For this review, take the finished solid that the model builds, in its own axes (mm). Face numbers are marked on the shaded views. A direction names the side the tool comes from. Coordinates: 2 decimals unless noted, no trailing zeros. Write each loop counter-clockwise with the first axis right and the second up, starting at its lowest first coordinate (ties: lowest second). Pieces come first, ordered by that corner, then holes.
```python
from build123d import *

# Parameters (mm, degrees)
SKETCH1_W           = 56.642
SKETCH1_H           = 32.258
BOSS_EXTRUDE1_DEPTH = 30.48
SHELL1_T            = -2.54
BOSS_EXTRUDE2_DEPTH = 6.35
FILLET2_R           = 2.54
FILLET3_R           = 2.54
CUT_EXTRUDE9_REACH  = 54.647
SKETCH10_W          = 22.86
SKETCH10_H          = 2.032
BOSS_EXTRUDE3_REACH = 46.623
SKETCH13_W          = 2.54
SKETCH13_H          = 3.81
SKETCH14_W          = 3.81
SKETCH14_H          = 1.27
BOSS_EXTRUDE4_DEPTH = 25.4
CUT_EXTRUDE10_DEPTH = 2.54
CUT_EXTRUDE11_REACH = 46.623
SKETCH16_W          = 9.652
SKETCH16_H          = 4.826
SKETCH11_R          = 1.27
CUT_EXTRUDE12_DEPTH = 9.398
MIRROR2_START       = 4.572
MIRROR2_OUTLINE_W   = 25.4
MIRROR2_OUTLINE_H   = 3.81
MIRROR2_DEPTH       = 2.54
SKETCH17_W          = 2.54
SKETCH17_H          = 3.81
CUT_EXTRUDE13_DEPTH = 23.368
SKETCH18_W          = 7.2898
SKETCH18_H          = 2.54
CUT_EXTRUDE14_DEPTH = 7.366
FILLET4_R           = 1.27
SKETCH19_W          = 2.54
SKETCH19_H          = 5.08
BOSS_EXTRUDE5_DEPTH = 2.54
CUT_EXTRUDE15_START = -23.368
SKETCH20_W          = 2.54
SKETCH20_H          = 3.81
CUT_EXTRUDE15_DEPTH = 23.368
SKETCH22_W          = 2.657331224
SKETCH22_H          = 5.08
CUT_EXTRUDE18_DEPTH = 6.858
SKETCH23_W          = 2.581688451
SKETCH23_H          = 6.7056
CUT_EXTRUDE19_DEPTH = 6.858
SKETCH24_W          = 4.254264989
SKETCH24_H          = 4.461970644
CUT_EXTRUDE20_DEPTH = 7.112


# Read off the part's stored shape, not the designer's step: Mirror2
with BuildPart() as part:
    # Sketch1 → Boss-Extrude1 (new body)
    with BuildSketch(Plane(origin=(0, 0, 0), x_dir=(1, 0, 0), z_dir=(0, 1, 0))):
        Rectangle(SKETCH1_W, SKETCH1_H)
    extrude(amount=BOSS_EXTRUDE1_DEPTH)

    # Shell1
    shell1_openings = [part.faces().sort_by_distance(p)[0] for p in [
        (0, 30.48, 0),
    ]]
    offset(amount=SHELL1_T, openings=shell1_openings, kind=Kind.INTERSECTION)

    # Sketch3 → Boss-Extrude2 (add)
    with BuildSketch(Plane(origin=(0, 30.48, 0), x_dir=(1, 0, 0), z_dir=(0, 1, 0))):
        with BuildLine():
            Line((-25.781, 13.589), (-25.781, 6.35))
            Line((-25.781, 6.35), (-23.9268, 6.35))
            ThreePointArc((-23.9268, 6.35), (-22.543840557, 6.922840557), (-21.971, 8.3058))
            Line((-21.971, 8.3058), (-21.971, 13.589))
            Line((-21.971, 13.589), (-25.781, 13.589))
        make_face()
        with BuildLine():
            Line((-21.971, -13.589), (-21.971, -8.3058))
            ThreePointArc((-21.971, -8.3058), (-22.543840557, -6.922840557), (-23.9268, -6.35))
            Line((-23.9268, -6.35), (-25.781, -6.35))
            Line((-25.781, -6.35), (-25.781, -13.589))
            Line((-25.781, -13.589), (-21.971, -13.589))
        make_face()
        with BuildLine():
            Line((25.781, 13.589), (19.2532, 13.589))
            Line((19.2532, 13.589), (19.2532, 5.969))
            ThreePointArc((19.2532, 5.969), (19.625174388, 5.070974388), (20.5232, 4.699))
            Line((20.5232, 4.699), (25.781, 4.699))
            Line((25.781, 4.699), (25.781, 13.589))
        make_face()
        with BuildLine():
            Line((25.781, -4.699), (25.781, -13.589))
            Line((25.781, -13.589), (19.2532, -13.589))
            Line((19.2532, -13.589), (19.2532, -5.969))
            ThreePointArc((19.2532, -5.969), (19.625174388, -5.070974388), (20.5232, -4.699))
            Line((20.5232, -4.699), (25.781, -4.699))
        make_face()
    extrude(amount=-BOSS_EXTRUDE2_DEPTH)

    # Fillet2
    fillet2_edges = [part.edges().sort_by_distance(p)[0] for p in [
        (28.321, 15.24, 16.129),
        (-28.321, 15.24, 16.129),
        (-28.321, 15.24, -16.129),
        (28.321, 15.24, -16.129),
    ]]
    fillet(fillet2_edges, radius=FILLET2_R)

    # Fillet3
    fillet3_edges = [part.edges().sort_by_distance(p)[0] for p in [
        (-25.781, 24.13, 9.9695),
        (-23.876, 24.13, 13.589),
        (22.5171, 24.13, 13.589),
        (25.781, 24.13, 9.144),
        (-23.876, 24.13, -13.589),
        (-25.781, 24.13, -9.9695),
        (22.5171, 24.13, -13.589),
        (25.781, 24.13, -9.144),
    ]]
    fillet(fillet3_edges, radius=FILLET3_R)

    # Cut-Extrude9: up to this face of the body (flat: up to its plane)
    cut_extrude9_end = Plane(part.part.faces().sort_by_distance((0, 15.24, 16.129))[0])
    # Sketch10 → Cut-Extrude9 (cut, up to the picked face)
    with BuildSketch(Plane(origin=(0, 0, -16.129), x_dir=(-1, 0, 0), z_dir=(0, 0, -1)), mode=Mode.PRIVATE) as cut_extrude9_sk1:
        with Locations((0, 3.556)):
            Rectangle(SKETCH10_W, SKETCH10_H)
    cut_extrude9_tool1 = split(extrude(cut_extrude9_sk1.sketch, amount=-CUT_EXTRUDE9_REACH, mode=Mode.PRIVATE), bisect_by=cut_extrude9_end, keep=Keep.BOTH, mode=Mode.PRIVATE)
    add(cut_extrude9_tool1.solids().sort_by(Axis((0, 3.556, -16.129), (0, 0, 1)))[0], mode=Mode.SUBTRACT)

    # Sketch13 → Boss-Extrude3 (add, up to next)
    with BuildSketch(Plane(origin=(0, 30.48, 0), x_dir=(1, 0, 0), z_dir=(0, 1, 0)), mode=Mode.PRIVATE) as boss_extrude3_sk1:
        with Locations((-13.97, -11.684)):
            Rectangle(SKETCH13_W, SKETCH13_H)
    boss_extrude3_tool1 = extrude(boss_extrude3_sk1.sketch, amount=-BOSS_EXTRUDE3_REACH, mode=Mode.PRIVATE) - part.part
    boss_extrude3 = boss_extrude3_tool1.solids().sort_by_distance((-13.97, 30.48, 11.684))[0]
    add(boss_extrude3)

    # Mirror1: Boss-Extrude3 across plane
    add(boss_extrude3.mirror(Plane(origin=(0, 0, 0), x_dir=(0, 0, 1), z_dir=(1, 0, 0))))

    # Sketch14 → Boss-Extrude4 (add)
    with BuildSketch(Plane.ZY.offset(-12.7)):
        with Locations((11.684, 5.207)):
            Rectangle(SKETCH14_W, SKETCH14_H)
    extrude(amount=BOSS_EXTRUDE4_DEPTH)

    # Sketch15 → Cut-Extrude10 (cut)
    with BuildSketch(Plane(origin=(0, 30.48, 0), x_dir=(1, 0, 0), z_dir=(0, 1, 0))):
        with BuildLine():
            Line((-25.781, 11.4046), (-25.781, 6.35))
            Line((-25.781, 6.35), (-23.9268, 6.35))
            ThreePointArc((-23.9268, 6.35), (-22.543840557, 6.922840557), (-21.971, 8.3058))
            Line((-21.971, 8.3058), (-21.971, 13.589))
            Line((-21.971, 13.589), (19.2532, 13.589))
            Line((19.2532, 13.589), (19.2532, 5.969))
            ThreePointArc((19.2532, 5.969), (19.625174388, 5.070974388), (20.5232, 4.699))
            Line((20.5232, 4.699), (25.781, 4.699))
            Line((25.781, 4.699), (25.781, -4.699))
            Line((25.781, -4.699), (20.5232, -4.699))
            ThreePointArc((20.5232, -4.699), (19.625174388, -5.070974388), (19.2532, -5.969))
            Line((19.2532, -5.969), (19.2532, -9.779))
            Line((19.2532, -9.779), (24.003, -9.779))
            ThreePointArc((24.003, -9.779), (25.799051224, -9.035051224), (26.543, -7.239))
            Line((26.543, -7.239), (26.543, -1.000588636))
            Line((26.543, -1.000588636), (26.543, 5.166188636))
            Line((26.543, 5.166188636), (26.543, 11.4046))
            ThreePointArc((26.543, 11.4046), (25.799051224, 13.200651224), (24.003, 13.9446))
            Line((24.003, 13.9446), (-23.241, 13.9446))
            ThreePointArc((-23.241, 13.9446), (-25.037051224, 13.200651224), (-25.781, 11.4046))
        make_face()
        with BuildLine():
            Line((-25.781, -6.35), (-25.781, -7.239))
            ThreePointArc((-25.781, -7.239), (-25.037051224, -9.035051224), (-23.241, -9.779))
            Line((-23.241, -9.779), (-21.971, -9.779))
            Line((-21.971, -9.779), (-21.971, -8.3058))
            ThreePointArc((-21.971, -8.3058), (-22.543840557, -6.922840557), (-23.9268, -6.35))
            Line((-23.9268, -6.35), (-25.781, -6.35))
        make_face()
    extrude(amount=-CUT_EXTRUDE10_DEPTH, mode=Mode.SUBTRACT)

    # Cut-Extrude11: up to this face of the body (flat: up to its plane)
    cut_extrude11_end = Plane(part.part.faces().sort_by_distance((28.321, 15.24, 0))[0])
    # Sketch16 → Cut-Extrude11 (cut, up to the picked face)
    with BuildSketch(Plane(origin=(0, 0, 0), x_dir=(0, 0, -1), z_dir=(1, 0, 0)), mode=Mode.PRIVATE) as cut_extrude11_sk1:
        with Locations((2.032, 26.797)):
            Rectangle(SKETCH16_W, SKETCH16_H)
    cut_extrude11_tool1 = split(extrude(cut_extrude11_sk1.sketch, amount=CUT_EXTRUDE11_REACH, mode=Mode.PRIVATE), bisect_by=cut_extrude11_end, keep=Keep.BOTH, mode=Mode.PRIVATE)
    add(cut_extrude11_tool1.solids().sort_by(Axis((0, 26.797, -2.032), (1, 0, 0)))[0], mode=Mode.SUBTRACT)

    # Sketch11 → Cut-Extrude12 (cut)
    with BuildSketch(Plane(origin=(0, 30.48, 0), x_dir=(1, 0, 0), z_dir=(0, 1, 0))):
        with Locations(Location((24.384, 11.5316, 0), (0, 0, 270))):
            Circle(SKETCH11_R)
        with Locations(Location((24.384, -6.2484, 0), (0, 0, 270))):
            Circle(SKETCH11_R)
    extrude(amount=-CUT_EXTRUDE12_DEPTH, mode=Mode.SUBTRACT)

    # Mirror2 outline → Mirror2 (add)
    with BuildSketch(Plane(origin=(0, 0, 0), x_dir=(1, 0, 0), z_dir=(0, 1, 0)).offset(MIRROR2_START)):
        with Locations((0, 11.684)):
            Rectangle(MIRROR2_OUTLINE_W, MIRROR2_OUTLINE_H)
        with Locations((0, -11.684)):
            Rectangle(MIRROR2_OUTLINE_W, MIRROR2_OUTLINE_H)
    extrude(amount=MIRROR2_DEPTH)

    # Sketch17 → Cut-Extrude13 (cut)
    with BuildSketch(Plane(origin=(0, 30.48, 0), x_dir=(1, 0, 0), z_dir=(0, 1, 0))):
        with Locations((-13.97, -11.684)):
            Rectangle(SKETCH17_W, SKETCH17_H)
    extrude(amount=-CUT_EXTRUDE13_DEPTH, mode=Mode.SUBTRACT)

    # Sketch18 → Cut-Extrude14 (cut)
    with BuildSketch(Plane(origin=(0, 27.94, 0), x_dir=(1, 0, 0), z_dir=(0, 1, 0))):
        with Locations((22.8981, 5.969)):
            Rectangle(SKETCH18_W, SKETCH18_H)
    extrude(amount=-CUT_EXTRUDE14_DEPTH, mode=Mode.SUBTRACT)

    # Fillet4
    fillet4_edges = [part.edges().sort_by_distance(p)[0] for p in [
        (27.432, 29.21, -6.858),
        (27.432, 24.384, -6.858),
        (27.051, 24.384, 2.794),
        (27.432, 29.21, 2.794),
    ]]
    fillet(fillet4_edges, radius=FILLET4_R)

    # Sketch19 → Boss-Extrude5 (add)
    with BuildSketch(Plane(origin=(0, 0, 13.589), x_dir=(-1, 0, 0), z_dir=(0, 0, -1))):
        with Locations((18.034, 9.652)):
            Rectangle(SKETCH19_W, SKETCH19_H)
    boss_extrude5 = extrude(amount=BOSS_EXTRUDE5_DEPTH)

    # Mirror3: Boss-Extrude5 across plane
    add(boss_extrude5.mirror(Plane.XY))

    # Sketch20 → Cut-Extrude15 (cut)
    with BuildSketch(Plane(origin=(0, 30.48, 0), x_dir=(1, 0, 0), z_dir=(0, 1, 0)).offset(CUT_EXTRUDE15_START)):
        with Locations((13.97, -11.684)):
            Rectangle(SKETCH20_W, SKETCH20_H)
    extrude(amount=CUT_EXTRUDE15_DEPTH, mode=Mode.SUBTRACT)

    # Sketch22 → Cut-Extrude18 (cut)
    with BuildSketch(Plane(origin=(0, 27.94, 0), x_dir=(1, 0, 0), z_dir=(0, 1, 0))):
        with Locations((20.581865612, -7.239)):
            Rectangle(SKETCH22_W, SKETCH22_H)
    extrude(amount=-CUT_EXTRUDE18_DEPTH, mode=Mode.SUBTRACT)

    # Sketch23 → Cut-Extrude19 (cut)
    with BuildSketch(Plane(origin=(0, 27.94, 0), x_dir=(1, 0, 0), z_dir=(0, 1, 0))):
        with Locations((20.544044226, 10.5918)):
            Rectangle(SKETCH23_W, SKETCH23_H)
    extrude(amount=-CUT_EXTRUDE19_DEPTH, mode=Mode.SUBTRACT)

    # Sketch24 → Cut-Extrude20 (cut)
    with BuildSketch(Plane(origin=(0, 27.94, 0), x_dir=(1, 0, 0), z_dir=(0, 1, 0))):
        with Locations((-23.653867506, 8.297478086)):
            Rectangle(SKETCH24_W, SKETCH24_H)
    extrude(amount=-CUT_EXTRUDE20_DEPTH, mode=Mode.SUBTRACT)


solid = part.part
```
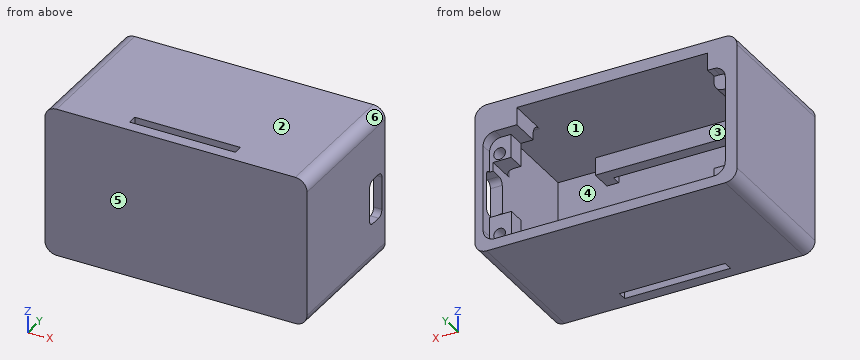
1) Consider section C-C (z = -8.5). Give the boundary of the cut face in (x, y).
2) For L1, parallel to X at y = 7, z = -13; L2, parallel to X at y = 16, z = 11; L3, parallel to Y at x = 11, z = 14, list the stretches that pass through material, from the lowest coordinate up.
3) Consider section D-D (x = 20.5). Give the boundary of the cut face in (y, z), then the cut area to 3 significant figures.
4) Tool access review of the marked faces 1 and 2: name each direction out of +Z, -Z, +X, -X, +Y, -Y from which nothing blocks a thin tool from reaching the whole face with its end or side.
5) Consider section A-A (y = 15). Give the boundary of the cut face in (x, z), then the cut area to 3 significant figures.
6) The part is to be moulded in two halves that separate along X. For the marked faces 3, 4, 5 and 6, say which applies: pulls with the +X half, pulls with the -X half, needs draft (parallel to the pull), parting line crosses it, or undercut.
7) Clearance check with flat-ended pins moving along their axes: P1, Ø2, axis at y = 4, z = 14.5, coming from the +X side; P2, Ø2.5, axis at x = 23.5, z = -10, coming from the +Y side; P3, Ø2, axis at x = -19, z = -5.5, coming from the +Y side; P4, Ø2.5, axis at x = 7.5, z = -12, coming from the +Y side. State where each tip first meets the part, or that it passes through.
8) Consider section B-B (x = -2). Give the boundary of the cut face in (y, z), then the cut area to 3 significant figures.
Results:
1. outline: (-28.32, 0) - (28.32, 0) - (28.32, 30.48) - (26.54, 30.48) - (26.54, 27.94) - (21.83, 27.94) - (21.83, 24.13) - (23.24, 24.13) arc R2.54 cw to (25.78, 21.59) - (25.78, 2.54) - (-25.78, 2.54) - (-25.78, 30.48) - (-28.32, 30.48) - close
2. L1: x = -28.32 to -25.78, -12.7 to 12.7, 25.78 to 28.32
2. L2: x = -28.32 to -25.78, 25.78 to 28.32
2. L3: y = 0 to 2.54, 4.57 to 30.48
3. outline: (0, -16.13) - (30.48, -16.13) - (30.48, -13.94) - (21.08, -13.94) - (21.08, -13.59) - (2.54, -13.59) - (2.54, 13.59) - (21.59, 13.59) arc R2.54 cw to (24.13, 11.05) - (24.13, 9.78) - (30.48, 9.78) - (30.48, 16.13) - (0, 16.13) - close
3. area: 246 mm2
4. face 1: none
4. face 2: +Z, +X, -X, +Y, -Y
5. outline: (-28.32, -13.59) arc R2.54 ccw to (-25.78, -16.13) - (25.78, -16.13) arc R2.54 ccw to (28.32, -13.59) - (28.32, 13.59) arc R2.54 ccw to (25.78, 16.13) - (-25.78, 16.13) arc R2.54 ccw to (-28.32, 13.59) - close; hole (-25.78, -13.59) - (25.78, -13.59) - (25.78, 13.59) - (-25.78, 13.59) - close
5. area: 420 mm2
6. face 3: undercut
6. face 4: undercut
6. face 5: needs draft
6. face 6: pulls with the +X half
7. P1: stops at x = 28.32
7. P2: stops at y = 27.94
7. P3: stops at y = 2.54
7. P4: stops at y = 7.11
8. outline: (0, -16.13) - (2.54, -16.13) - (2.54, 16.13) - (0, 16.13) - close; (4.57, -16.13) - (30.48, -16.13) - (30.48, -13.94) - (27.94, -13.94) - (27.94, -13.59) - (7.11, -13.59) - (7.11, -9.78) - (4.57, -9.78) - close; (4.57, 9.78) - (7.11, 9.78) - (7.11, 13.59) - (30.48, 13.59) - (30.48, 16.13) - (4.57, 16.13) - close
8. area: 232 mm2
